```python
from build123d import *

# Parameters (mm, degrees)
F0_W         = 82
F0_H         = 9.9
F1_DEPTH     = 20
F2_T         = -2
F3_DEPTH     = 2
F4_DEPTH     = 5
F6_R         = 1.3971487494
F5_R         = 1.9718048452
F7_DEPTH     = 74
F8_W         = 55.0399487838
F8_H         = 7.4755754322
F9_DEPTH     = 2
F10_T1_DEPTH = 2
F11_R        = 3
F12_W        = 1.8215961754
F12_H        = 3.4220837988
F13_DEPTH    = 1
F14_T4_DEPTH = 3.4220837988
F14_T9_DEPTH = 3.4220837988
F15_R        = 0.7
F16_W        = 0.433061509
F16_H        = 3.4220837988
F16_W_2      = 1.2856977906
F16_W_3      = 0.4418755459
F17_DEPTH    = 73
F19_DEPTH    = 10
F20_DEPTH    = 5


# Not quite as in the source:
# - a fillet or chamfer that OpenCascade refuses, or shapes differently, is made with other operations: its cross-section is extruded or revolved along the edge and cut away or added
# - a feature of the source that left no trace in its solid (it failed there, or was rolled back) is left out


with BuildPart() as f1:
    # F0 (on Top) → F1 (new body)
    with BuildSketch(Plane.XY):
        with Locations((-34.3298178315, -49.909187454)):
            Rectangle(F0_W, F0_H)
    extrude(amount=F1_DEPTH)

    # F2
    f2_openings = [f1.faces().sort_by_distance(p)[0] for p in [
        (-34.329818, -54.859187, 10),
    ]]
    offset(amount=F2_T, openings=f2_openings)

    # F3 (cut): a face of the model
    f3_faces = [f1.faces().sort_by_distance(p)[0] for p in [
        (-34.3298178315, -50.909187454, 2),
    ]]
    extrude(f3_faces, amount=-F3_DEPTH, mode=Mode.SUBTRACT)

    # F4 (add): a face of the model
    f4_faces = [f1.faces().sort_by_distance(p)[0] for p in [
        (4.6701821685, -50.909187454, 9),
    ]]
    extrude(f4_faces, amount=F4_DEPTH)

    # F6 (on face) + F5 (on face) → F7 (join)
    with BuildSketch(Plane(origin=(-0.3298178315, 0, 0), x_dir=(0, -1, 0), z_dir=(-1, 0, 0))):
        with Locations((50.704728812, 13.591603376)):
            Circle(F6_R)
    with BuildSketch(Plane(origin=(-0.3298178315, 0, 0), x_dir=(0, -1, 0), z_dir=(-1, 0, 0))):
        with Locations((50.909187454, 2.9176021926)):
            Circle(F5_R)
    extrude(amount=F7_DEPTH)

    # F8 (on face) → F9 (cut)
    with BuildSketch(Plane.XZ.offset(46.959187454)):
        with Locations((-38.2777568884, 9.5675773919)):
            Rectangle(F8_W, F8_H)
    extrude(amount=-F9_DEPTH, mode=Mode.SUBTRACT)

    # F10: fillet of radius 5 on 4 edges, made by hand

    # F10_s2 → F10_t1 (join)
    with BuildSketch(Plane.XZ.offset(44.959187454)):
        with BuildLine():
            ThreePointArc((-15.7577824965, 5.8297896758), (-12.2222485906, 7.2942557698), (-10.7577824965, 10.8297896758))
            Line((-10.7577824965, 10.8297896758), (-10.7577824965, 5.8297896758))
            Line((-10.7577824965, 5.8297896758), (-15.7577824965, 5.8297896758))
        make_face()
        with BuildLine():
            ThreePointArc((-65.7977312803, 10.8297896758), (-64.3332651863, 7.2942557698), (-60.7977312803, 5.8297896758))
            Line((-60.7977312803, 5.8297896758), (-65.7977312803, 5.8297896758))
            Line((-65.7977312803, 5.8297896758), (-65.7977312803, 10.8297896758))
        make_face()
        with BuildLine():
            ThreePointArc((-60.7977312803, 13.305365108), (-64.3332651863, 11.8408990139), (-65.7977312803, 8.305365108))
            Line((-65.7977312803, 8.305365108), (-65.7977312803, 13.305365108))
            Line((-65.7977312803, 13.305365108), (-60.7977312803, 13.305365108))
        make_face()
        with BuildLine():
            ThreePointArc((-15.7577824965, 13.305365108), (-12.2222485906, 11.8408990139), (-10.7577824965, 8.305365108))
            Line((-10.7577824965, 8.305365108), (-10.7577824965, 13.305365108))
            Line((-10.7577824965, 13.305365108), (-15.7577824965, 13.305365108))
        make_face()
    extrude(amount=F10_T1_DEPTH)

    # F11
    f11_edges = [f1.edges().sort_by_distance(p)[0] for p in [
        (-10.919723, -45.959187, 9.567577),
        (-65.635791, -45.959187, 9.567577),
    ]]
    fillet(f11_edges, radius=F11_R)

    # F12 (on face) → F13 (join)
    with BuildSketch(Plane(origin=(-0.3298178315, 0, 0), x_dir=(0, -1, 0), z_dir=(-1, 0, 0))):
        with Locations((51.1129107326, 7.6496207621)):
            Rectangle(F12_W, F12_H)
    extrude(amount=F13_DEPTH)

    # F14: fillet of radius 2 on 2 edges, made by hand


with BuildPart() as f14_tool2:
    # F14_s3 → F14_t4 (new body)
    with BuildSketch(Plane.XY.offset(5.9385788627)):
        with BuildLine():
            ThreePointArc((0.6701821685, -52.0237088203), (-0.7440313939, -51.4379223827), (-1.3298178315, -50.0237088203))
            Line((-1.3298178315, -50.0237088203), (-1.3698178315, -50.0237088203))
            Line((-1.3698178315, -50.0237088203), (-1.3698178315, -52.0637088203))
            Line((-1.3698178315, -52.0637088203), (0.6701821685, -52.0637088203))
            Line((0.6701821685, -52.0637088203), (0.6701821685, -52.0237088203))
        make_face()
    extrude(amount=F14_T4_DEPTH)

    split(bisect_by=Plane.YZ.offset(-0.3298178315), keep=Keep.BOTTOM)


with BuildPart() as f1_1:
    add(f1.part)

    # F14_t1: cut F14_tool2
    add(f14_tool2.part, mode=Mode.SUBTRACT)


with BuildPart() as f14_tool7:
    # F14_s8 → F14_t9 (new body)
    with BuildSketch(Plane.XY.offset(9.3606626615)):
        with BuildLine():
            ThreePointArc((0.6701821685, -50.2021126449), (-0.7440313939, -50.7878990825), (-1.3298178315, -52.2021126449))
            Line((-1.3298178315, -52.2021126449), (-1.3698178315, -52.2021126449))
            Line((-1.3698178315, -52.2021126449), (-1.3698178315, -50.1621126449))
            Line((-1.3698178315, -50.1621126449), (0.6701821685, -50.1621126449))
            Line((0.6701821685, -50.1621126449), (0.6701821685, -50.2021126449))
        make_face()
    extrude(amount=-F14_T9_DEPTH)

    split(bisect_by=Plane.YZ.offset(-0.3298178315), keep=Keep.BOTTOM)


with BuildPart() as f1_2:
    add(f1_1.part)

    # F14_t6: cut F14_tool7
    add(f14_tool7.part, mode=Mode.SUBTRACT)

    # F15
    f15_edges = [f1_2.edges().sort_by_distance(p)[0] for p in [
        (-1.007208, -51.112911, 7.649621),
    ]]
    fillet(f15_edges, radius=F15_R)

    # F16 (on face) → F17 (join)
    with BuildSketch(Plane(origin=(-0.3298178315, 0, 0), x_dir=(0, -1, 0), z_dir=(-1, 0, 0))):
        with Locations((50.2535310828, 7.6496207621)):
            Rectangle(F16_W, F16_H)
        with Locations((51.1129107326, 7.6496207621)):
            Rectangle(F16_W_2, F16_H)
        with Locations((51.9766974008, 7.6496207621)):
            Rectangle(F16_W_3, F16_H)
    extrude(amount=F17_DEPTH)

    # F19 (add): a face of the model
    f19_faces = [f1_2.faces().sort_by_distance(p)[0] for p in [
        (-75.3298178315, -49.909187454, 10),
    ]]
    extrude(f19_faces, amount=F19_DEPTH)

    # F20 (cut): a face of the model
    f20_faces = [f1_2.faces().sort_by_distance(p)[0] for p in [
        (-73.3298178315, -50.9067397847, 9.4818900009),
    ]]
    extrude(f20_faces, amount=-F20_DEPTH, mode=Mode.SUBTRACT)


solid = f1_2.part
```
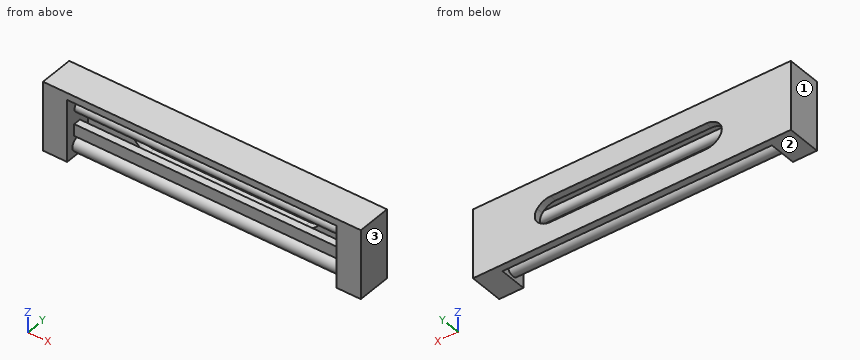
Source: CAD feature listing. Evaluate the final solid. Frame: model axes, mm. Face numbers are marked on the shaded views. Give positions to 0.01 mm unless a question says otherwise; leave off trailing zeros. Loops run counter-clockwise (first coordinate to the right, second up) from the corner with the lowest first, then second, coordinate; pieces in that order, holes last. Notation, with made-up numbers: (11.5, 10.5) - (60.5, 10.5) arc R32 ccw to (60.5, 49.5) - close; hole circle Ø6 at (46.5, 41.25). An arc over 180 degrees is marked (long way). Use CSV: the item, a comma, the result in double quotes. Start each with the question number.
1. Section A-A (x = -63.5). Output: boundary loops of the cut face in (y, z).
2. Section C-C (x = -7). Output: boundary loops of the cut face in (y, z), then the cut area to 3 significant figures.
3. Pin query (flat end, axial travel): pin 1 (2.5 mm diameter, centred on x = -45.5, y = -51.5, fed in from -Z); pin 2 (5.5 mm diameter, centred on x = -37.5, z = 9.5, fed in from -Y); pin 3 (1 mm diameter, centred on x = -49.5, z = 7.5, fed in from +Y); pin 4 (1 mm diameter, centred on x = -46, z = 11.5, fed in from -Y). Return the tip coordinate at first contact, or that it passes through.
4. Section B-B (z = 15.75). Output: boundary loops of the cut face in (x, y).
5. Section D-D (x = -53). Output: boundary loops of the cut face in (y, z), then the cut area to 3 significant figures.
6. Ray query, L1, parallel to X at y = -51.25, z = 10.5; L2, parallel to Y at x = -4.5, z = 7.5; L3, parallel to Z at x = -5.5, y = -50.75. Return the intervals inside material, ascending.
7. Draft query along X for the marked faces 1, 2 and 3. Return one class per face: +X half, -X half, draft (parallel to the pull), parting line (faces both ways), or undercut.
Response:
1,outline,"(-54.86, 18) - (-46.96, 18) - (-46.96, 12.51) - (-44.96, 12.51) - (-44.96, 20) - (-54.86, 20) - close; circle Ø3.94 at (-50.91, 2.92); (-52.2, 5.94) - (-50.04, 5.94) - (-50.04, 9.36) - (-52.2, 9.36) - close; circle Ø2.79 at (-50.7, 13.59); (-46.96, 0) - (-44.96, 0) - (-44.96, 6.62) - (-46.96, 6.62) - close"
2,outline,"(-54.86, 18) - (-46.96, 18) - (-46.96, 0) - (-44.96, 0) - (-44.96, 20) - (-54.86, 20) - close; circle Ø3.94 at (-50.91, 2.92); (-52.2, 5.94) - (-50.04, 5.94) - (-50.04, 9.36) - (-52.2, 9.36) - close; circle Ø2.79 at (-50.7, 13.59)"
2,area,"81.5 mm²"
3,pin 1,"z = 0.95"
3,pin 2,"y = -52.2"
3,pin 3,"y = -50.04"
3,pin 4,"through"
4,outline,"(-85.33, -54.86) - (-78.33, -54.86) - (-78.33, -46.96) - (-0.33, -46.96) - (-0.33, -54.86) - (6.67, -54.86) - (6.67, -44.96) - (-85.33, -44.96) - close"
5,outline,"(-54.86, 18) - (-46.96, 18) - (-46.96, 13.31) - (-44.96, 13.31) - (-44.96, 20) - (-54.86, 20) - close; circle Ø3.94 at (-50.91, 2.92); (-52.2, 5.94) - (-50.04, 5.94) - (-50.04, 9.36) - (-52.2, 9.36) - close; circle Ø2.79 at (-50.7, 13.59); (-46.96, 0) - (-44.96, 0) - (-44.96, 5.83) - (-46.96, 5.83) - close"
5,area,"66.6 mm²"
6,L1,"-85.33 to -78.33, -0.33 to 6.67"
6,L2,"-52.2 to -50.04, -46.96 to -44.96"
6,L3,"0.95 to 4.88, 5.94 to 9.36, 12.2 to 14.99, 18 to 20"
7,face 1,"-X half"
7,face 2,"draft"
7,face 3,"+X half"
